```python
from build123d import *

# Parameters (mm, degrees)
SKETCH1_W                                   = 95.169284227
SKETCH1_H                                   = 71.949644858
BOSS_EXTRUDE1_DEPTH                         = 10
CBORE_FOR_3_BINDING_HEAD_MACHINE_SC_2_COUNT = 2
CBORE_FOR_3_BINDING_HEAD_MACHINE_SC_2_PITCH = 54.707018707
CBORE_FOR_3_BINDING_HEAD_MACHINE_SC_3_COUNT = 2
CBORE_FOR_3_BINDING_HEAD_MACHINE_SC_3_PITCH = 73.126317411
CBORE_FOR_3_BINDING_HEAD_MACHINE_SC_4_COUNT = 2
CBORE_FOR_3_BINDING_HEAD_MACHINE_SC_4_PITCH = 91.332818695


with BuildPart() as part:
    # Sketch1 → Boss-Extrude1 (new body)
    with BuildSketch(Plane(origin=(0, 0, 0), x_dir=(1, 0, 0), z_dir=(0, 1, 0))):
        with Locations((47.584642114, 35.974822429)):
            Rectangle(SKETCH1_W, SKETCH1_H)
    extrude(amount=BOSS_EXTRUDE1_DEPTH)

    # Sketch3 → CBORE for #3 Binding Head Machine Screw1 (revolve, cut)
    with BuildSketch(Plane(origin=(11.17, 10, -63.944240186), x_dir=(0, 0, 1), z_dir=(1, 0, 0))):
        Polygon((0, 0), (0, 10), (1.397, 10), (1.397, 1.4986), (2.97688, 1.4986), (2.97688, 0.635), (3.61188, 0), align=None)
    cbore_for_3_binding_head_machine_screw1 = revolve(axis=Axis((11.17, 16.35, -63.944240186), (0, -1, 0)), mode=Mode.SUBTRACT)

    # CBORE for _3 Binding Head Machine Sc 2: CBORE for #3 Binding Head Machine Screw1 ×2
    with Locations(*[(0, 0, i * CBORE_FOR_3_BINDING_HEAD_MACHINE_SC_2_PITCH) for i in range(1, CBORE_FOR_3_BINDING_HEAD_MACHINE_SC_2_COUNT)]):
        add(cbore_for_3_binding_head_machine_screw1, mode=Mode.SUBTRACT)

    # CBORE for _3 Binding Head Machine Sc 3: CBORE for #3 Binding Head Machine Screw1 ×2
    with Locations(*[Vector(0.9999999980255075, 0, 6.284095007611635e-05) * (i * CBORE_FOR_3_BINDING_HEAD_MACHINE_SC_3_PITCH) for i in range(1, CBORE_FOR_3_BINDING_HEAD_MACHINE_SC_3_COUNT)]):
        add(cbore_for_3_binding_head_machine_screw1, mode=Mode.SUBTRACT)

    # CBORE for _3 Binding Head Machine Sc 4: CBORE for #3 Binding Head Machine Screw1 ×2
    with Locations(*[Vector(0.8006979380692495, 0, 0.5990682865681111) * (i * CBORE_FOR_3_BINDING_HEAD_MACHINE_SC_4_PITCH) for i in range(1, CBORE_FOR_3_BINDING_HEAD_MACHINE_SC_4_COUNT)]):
        add(cbore_for_3_binding_head_machine_screw1, mode=Mode.SUBTRACT)


solid = part.part
```
CAD build for the part. Positions are in the model's coordinates, mm. A direction names the side the tool comes from. Round coordinates to 2 decimals unless told otherwise and drop trailing zeros. Loops run counter-clockwise (first coordinate to the right, second up) from the corner with the lowest first, then second, coordinate; pieces in that order, holes last. Notation, with made-up numbers: M 37.5,48.25 L 49.5,48.25 A15 cw 49.5,66.25 Z; hole C 6.25,28 d11. An arc over 180 degrees is marked long. Return JSON: item names as keys, results as strings. Group by question number.
(1) Mould opens along X. For faces 3 (the flat face through (95.169, 5, -35)), 4 (the flat face through (47, 0, -36)), 5 (the cylindrical face through (14.076, 8.939, -9.883)) say: +X half, -X half, draft (parallel to the pull), parting line (faces both ways), or undercut.
(2) Wall check: probe 1 along X at (y, z) = (6.25, -9); probe 2 along X at (y, z) = (1.75, -8); probe 3 along Z at (x, y) = (11.17, 6.75). Give the ranges that are in metal, low to high. Write a range as [from, to].
(3) Saw through at A-A, the plane x = 11.17. List the corners of the cut face in (y, z) (3 decimals).
(4) Tool access for faces 1 (the flat face through (47, 5, -71.95)), 2 (the cylindrical face through (12.31, 8.939, -61.194)): list every direction of +Z, -Z, +X, -X, +Y, -Y with a clear straight run to the whole face (end or side of a thin tool).
(5) Drop flat-ended pins along their axis: P1, Ø1.8, axis at x = 12, z = -65, coming from the +Y side; P2, Ø7, axis at x = 11.17, z = -63.94, coming from the +Y side. Give the stop position or say it passes through.
Answer list:
{
 "1": {"face 3": "+X half", "face 4": "draft", "face 5": "undercut"},
 "2": {"probe 1": "[0, 9.79], [12.55, 82.92], [85.68, 95.17]", "probe 2": "[0, 10.52], [11.82, 83.64], [84.96, 95.17]", "probe 3": "[-71.95, -65.34], [-62.55, -10.63], [-7.84, 0]"},
 "3": {"outline": "M 0,-71.95 L 10,-71.95 L 10,-67.556 L 9.365,-66.921 L 8.501,-66.921 L 8.501,-65.341 L 0,-65.341 Z; M 0,-62.547 L 8.501,-62.547 L 8.501,-60.967 L 9.365,-60.967 L 10,-60.332 L 10,-12.849 L 9.365,-12.214 L 8.501,-12.214 L 8.501,-10.634 L 0,-10.634 Z; M 0,-7.84 L 8.501,-7.84 L 8.501,-6.26 L 9.365,-6.26 L 10,-5.625 L 10,0 L 0,0 Z"},
 "4": {"face 1": "-Z, +X, -X, +Y, -Y", "face 2": "+Y"},
 "5": {"P1": "y = 8.5", "P2": "y = 9.89"}
}
